```python
from build123d import *

# Parameters (mm, degrees)
SKETCH1_R           = 1.5
BOSS_EXTRUDE1_DEPTH = 3
SCALE1_SCALE        = 0.888888889


with BuildPart() as part:
    # Sketch1 → Boss-Extrude1 (new body)
    with BuildSketch(Plane(origin=(0, 0, 0), x_dir=(1, 0, 0), z_dir=(0, 1, 0))):
        with BuildLine():
            Line((20.893657446, 4), (2.081641936, 4))
            ThreePointArc((2.081641936, 4), (2.861028333, 4.588201733), (3.521749436, 5.30713988))
            ThreePointArc((3.521749436, 5.30713988), (3.405395609, 5.596745198), (3.282888305, 5.883801663))
            ThreePointArc((3.282888305, 5.883801663), (1.93527598, 5.894040025), (0.627094961, 5.57027124))
            ThreePointArc((0.627094961, 5.57027124), (0.366286148, 6.046375), (0.084372603, 6.510293938))
            ThreePointArc((0.084372603, 6.510293938), (1.018855105, 7.48132754), (1.683794586, 8.65351323))
            ThreePointArc((1.683794586, 8.65351323), (1.496450048, 8.903135899), (1.303821399, 9.148703928))
            ThreePointArc((1.303821399, 9.148703928), (-0.000522033, 8.809805691), (-1.180330337, 8.158486898))
            ThreePointArc((-1.180330337, 8.158486898), (-1.555477026, 8.550865528), (-1.947855656, 8.926012217))
            ThreePointArc((-1.947855656, 8.926012217), (-1.296536862, 10.105820521), (-0.957638625, 11.410163953))
            ThreePointArc((-0.957638625, 11.410163953), (-1.203206655, 11.602792602), (-1.452829324, 11.79013714))
            ThreePointArc((-1.452829324, 11.79013714), (-2.625015014, 11.125197659), (-3.596048616, 10.190715157))
            ThreePointArc((-3.596048616, 10.190715157), (-4.059967554, 10.472628702), (-4.536071314, 10.733437515))
            ThreePointArc((-4.536071314, 10.733437515), (-4.212302529, 12.041618533), (-4.222540891, 13.389230859))
            ThreePointArc((-4.222540891, 13.389230859), (-4.509597355, 13.511738163), (-4.799202674, 13.62809199))
            ThreePointArc((-4.799202674, 13.62809199), (-5.759348103, 12.682425791), (-6.455432668, 11.528463019))
            ThreePointArc((-6.455432668, 11.528463019), (-6.976508546, 11.680699536), (-7.503891752, 11.809396783))
            ThreePointArc((-7.503891752, 11.809396783), (-7.529737283, 13.156800143), (-7.888414517, 14.455843809))
            ThreePointArc((-7.888414517, 14.455843809), (-8.197396993, 14.499881098), (-8.507248835, 14.537314892))
            ThreePointArc((-8.507248835, 14.537314892), (-9.18992168, 13.375367565), (-9.563620196, 12.080565177))
            ThreePointArc((-9.563620196, 12.080565177), (-10.106342554, 12.09275), (-10.649064912, 12.080565177))
            ThreePointArc((-10.649064912, 12.080565177), (-11.022763428, 13.375367565), (-11.705436272, 14.537314892))
            ThreePointArc((-11.705436272, 14.537314892), (-12.015288115, 14.499881098), (-12.324270591, 14.455843809))
            ThreePointArc((-12.324270591, 14.455843809), (-12.682947825, 13.156800143), (-12.708793355, 11.809396783))
            ThreePointArc((-12.708793355, 11.809396783), (-13.236176561, 11.680699536), (-13.757252439, 11.528463019))
            ThreePointArc((-13.757252439, 11.528463019), (-14.453337005, 12.682425791), (-15.413482434, 13.62809199))
            ThreePointArc((-15.413482434, 13.62809199), (-15.703087752, 13.511738163), (-15.990144217, 13.389230859))
            ThreePointArc((-15.990144217, 13.389230859), (-16.000382579, 12.041618533), (-15.676613793, 10.733437515))
            ThreePointArc((-15.676613793, 10.733437515), (-16.152717554, 10.472628702), (-16.616636492, 10.190715157))
            ThreePointArc((-16.616636492, 10.190715157), (-17.587670094, 11.125197659), (-18.759855783, 11.79013714))
            ThreePointArc((-18.759855783, 11.79013714), (-19.009478453, 11.602792602), (-19.255046482, 11.410163953))
            ThreePointArc((-19.255046482, 11.410163953), (-18.916148245, 10.105820521), (-18.264829452, 8.926012217))
            ThreePointArc((-18.264829452, 8.926012217), (-18.657208082, 8.550865528), (-19.032354771, 8.158486898))
            ThreePointArc((-19.032354771, 8.158486898), (-20.212163074, 8.809805691), (-21.516506507, 9.148703928))
            ThreePointArc((-21.516506507, 9.148703928), (-21.709135156, 8.903135899), (-21.896479694, 8.65351323))
            ThreePointArc((-21.896479694, 8.65351323), (-21.231540213, 7.48132754), (-20.297057711, 6.510293938))
            ThreePointArc((-20.297057711, 6.510293938), (-20.578971255, 6.046375), (-20.839780068, 5.57027124))
            ThreePointArc((-20.839780068, 5.57027124), (-22.147961087, 5.894040025), (-23.495573413, 5.883801663))
            ThreePointArc((-23.495573413, 5.883801663), (-23.618080717, 5.596745198), (-23.734434544, 5.30713988))
            ThreePointArc((-23.734434544, 5.30713988), (-22.788768345, 4.346994451), (-21.634805572, 3.650909885))
            ThreePointArc((-21.634805572, 3.650909885), (-21.78704209, 3.129834008), (-21.915739337, 2.602450802))
            ThreePointArc((-21.915739337, 2.602450802), (-23.263142697, 2.576605271), (-24.562186363, 2.217928037))
            ThreePointArc((-24.562186363, 2.217928037), (-24.606223651, 1.908945561), (-24.643657446, 1.599093719))
            ThreePointArc((-24.643657446, 1.599093719), (-23.481710119, 0.916420874), (-22.186907731, 0.542722358))
            ThreePointArc((-22.186907731, 0.542722358), (-22.199092554, 0), (-22.186907731, -0.542722358))
            ThreePointArc((-22.186907731, -0.542722358), (-23.481710119, -0.916420874), (-24.643657446, -1.599093719))
            ThreePointArc((-24.643657446, -1.599093719), (-24.606223651, -1.908945561), (-24.562186363, -2.217928037))
            ThreePointArc((-24.562186363, -2.217928037), (-23.263142697, -2.576605271), (-21.915739337, -2.602450802))
            ThreePointArc((-21.915739337, -2.602450802), (-21.78704209, -3.129834008), (-21.634805572, -3.650909885))
            ThreePointArc((-21.634805572, -3.650909885), (-22.788768345, -4.346994451), (-23.734434544, -5.30713988))
            ThreePointArc((-23.734434544, -5.30713988), (-23.618080717, -5.596745198), (-23.495573413, -5.883801663))
            ThreePointArc((-23.495573413, -5.883801663), (-22.147961087, -5.894040025), (-20.839780068, -5.57027124))
            ThreePointArc((-20.839780068, -5.57027124), (-20.578971255, -6.046375), (-20.297057711, -6.510293938))
            ThreePointArc((-20.297057711, -6.510293938), (-21.231540213, -7.48132754), (-21.896479694, -8.65351323))
            ThreePointArc((-21.896479694, -8.65351323), (-21.709135156, -8.903135899), (-21.516506507, -9.148703928))
            ThreePointArc((-21.516506507, -9.148703928), (-20.212163074, -8.809805691), (-19.032354771, -8.158486898))
            ThreePointArc((-19.032354771, -8.158486898), (-18.657208082, -8.550865528), (-18.264829452, -8.926012217))
            ThreePointArc((-18.264829452, -8.926012217), (-18.916148245, -10.105820521), (-19.255046482, -11.410163953))
            ThreePointArc((-19.255046482, -11.410163953), (-19.009478453, -11.602792602), (-18.759855783, -11.79013714))
            ThreePointArc((-18.759855783, -11.79013714), (-17.587670094, -11.125197659), (-16.616636492, -10.190715157))
            ThreePointArc((-16.616636492, -10.190715157), (-16.152717554, -10.472628702), (-15.676613793, -10.733437515))
            ThreePointArc((-15.676613793, -10.733437515), (-16.000382579, -12.041618533), (-15.990144217, -13.389230859))
            ThreePointArc((-15.990144217, -13.389230859), (-15.703087752, -13.511738163), (-15.413482434, -13.62809199))
            ThreePointArc((-15.413482434, -13.62809199), (-14.453337005, -12.682425791), (-13.757252439, -11.528463019))
            ThreePointArc((-13.757252439, -11.528463019), (-13.236176561, -11.680699536), (-12.708793355, -11.809396783))
            ThreePointArc((-12.708793355, -11.809396783), (-12.682947825, -13.156800143), (-12.324270591, -14.455843809))
            ThreePointArc((-12.324270591, -14.455843809), (-12.015288115, -14.499881098), (-11.705436272, -14.537314892))
            ThreePointArc((-11.705436272, -14.537314892), (-11.022763428, -13.375367565), (-10.649064912, -12.080565177))
            ThreePointArc((-10.649064912, -12.080565177), (-10.106342554, -12.09275), (-9.563620196, -12.080565177))
            ThreePointArc((-9.563620196, -12.080565177), (-9.18992168, -13.375367565), (-8.507248835, -14.537314892))
            ThreePointArc((-8.507248835, -14.537314892), (-8.197396993, -14.499881098), (-7.888414517, -14.455843809))
            ThreePointArc((-7.888414517, -14.455843809), (-7.529737283, -13.156800143), (-7.503891752, -11.809396783))
            ThreePointArc((-7.503891752, -11.809396783), (-6.976508546, -11.680699536), (-6.455432668, -11.528463019))
            ThreePointArc((-6.455432668, -11.528463019), (-5.759348103, -12.682425791), (-4.799202674, -13.62809199))
            ThreePointArc((-4.799202674, -13.62809199), (-4.509597355, -13.511738163), (-4.222540891, -13.389230859))
            ThreePointArc((-4.222540891, -13.389230859), (-4.212302529, -12.041618533), (-4.536071314, -10.733437515))
            ThreePointArc((-4.536071314, -10.733437515), (-4.059967554, -10.472628702), (-3.596048616, -10.190715157))
            ThreePointArc((-3.596048616, -10.190715157), (-2.625015014, -11.125197659), (-1.452829324, -11.79013714))
            ThreePointArc((-1.452829324, -11.79013714), (-1.203206655, -11.602792602), (-0.957638625, -11.410163953))
            ThreePointArc((-0.957638625, -11.410163953), (-1.296536862, -10.105820521), (-1.947855656, -8.926012217))
            ThreePointArc((-1.947855656, -8.926012217), (-1.555477026, -8.550865528), (-1.180330337, -8.158486898))
            ThreePointArc((-1.180330337, -8.158486898), (-0.000522033, -8.809805691), (1.303821399, -9.148703928))
            ThreePointArc((1.303821399, -9.148703928), (1.496450048, -8.903135899), (1.683794586, -8.65351323))
            ThreePointArc((1.683794586, -8.65351323), (1.018855105, -7.48132754), (0.084372603, -6.510293938))
            ThreePointArc((0.084372603, -6.510293938), (0.366286148, -6.046375), (0.627094961, -5.57027124))
            ThreePointArc((0.627094961, -5.57027124), (1.93527598, -5.894040025), (3.282888305, -5.883801663))
            ThreePointArc((3.282888305, -5.883801663), (3.405395609, -5.596745198), (3.521749436, -5.30713988))
            ThreePointArc((3.521749436, -5.30713988), (2.861028333, -4.588201733), (2.081641936, -4))
            Line((2.081641936, -4), (20.893657446, -4))
            ThreePointArc((20.893657446, -4), (24.893657446, 0), (20.893657446, 4))
        make_face()
        with Locations(Location((-10.106342554, 0, 0), (0, 0, 270))):
            Circle(SKETCH1_R, mode=Mode.SUBTRACT)
        with Locations(Location((20.893657446, 0, 0), (0, 0, 270))):
            Circle(SKETCH1_R, mode=Mode.SUBTRACT)
    extrude(amount=BOSS_EXTRUDE1_DEPTH)


with BuildPart() as part_1:
    # Scale1: scaled about (-4.801213178, 1.5, 0)
    add(part.part.scale(SCALE1_SCALE).moved(Location((-0.533468131, 0.166666667, 0))))


solid = part_1.part
```
Work out the finished part from the listing and answer in its coordinate system (mm). A direction names the side the tool comes from. Coordinates: 2 decimals unless noted, no trailing zeros. Write each loop counter-clockwise with the first axis right and the second up, starting at its lowest first coordinate (ties: lowest second). Pieces come first, ordered by that corner, then holes.
Q1. A cutting plane is placed at A-A, the plane z = 0. Give the vertices of the cut face in (x, y), then the cut area to 3 significant figures.
Q2. Determine the mould class of faces 5 (the face through (-9.52, 1.48, 10.75)), 6 (the face through (-2.85, 1.48, -9.9)), 7 (the face through (-0.205, 1.481, -5.369)) for opening direction Z: released by +Z, released by -Z, zero draft, split by the parting line, or undercut.
Q3. Which of the six approach directions +Z, -Z, +X, -X, +Y, -Y give full straight-line access (tool end or side, diameter ignored) to faces 1 (the face through (-8.71, 1.48, 11.87)), 2 (the face through (-16.153, 1.481, -9.879)), 3 (the face through (-14.89, 1.48, -9.31)), 4 (the face through (0.362, 1.481, -6.637))?
Q4. Find the intervals of material crossed by line 1 (X direction, y = 1.2, z = 0); line 2 (Z direction, x = 0, y = 2.35); line 3 (X direction, y = 2.05, z = 7.5), in increasing order.
Q5. A cutting plane is placed at B-B, the plane y = 1.4. State how many separate pieces and enclosed holes the cut face has, then the cut area to 3 significant figures.
Q6. This flat-tipped pin is pushed along its axis until it touches: pin 1 Ø1.3 at (x, y) = (8.5, 2) entering from +Z. Where does it stop, or does it pass through?
Findings below:
1. outline: (-20.27, 0.17) - (-10.85, 0.17) - (-10.85, 2.83) - (-20.27, 2.83) - close; (-8.18, 0.17) - (16.71, 0.17) - (16.71, 2.83) - (-8.18, 2.83) - close; (19.37, 0.17) - (21.59, 0.17) - (21.59, 2.83) - (19.37, 2.83) - close
1. area: 97.4 mm2
2. face 5: released by +Z
2. face 6: released by -Z
2. face 7: undercut
3. face 1: +Z, +Y, -Y
3. face 2: -Z, +Y, -Y
3. face 3: +Y, -Y
3. face 4: +X, +Y, -Y
4. line 1: x = -20.27 to -10.85, -8.18 to 16.71, 19.37 to 21.59
4. line 2: z = -8.01 to -6.21, -5 to 5, 6.21 to 8.01
4. line 3: x = -19.91 to -17.83, -17.22 to -1.82, -1.21 to 0.88
5. separate pieces: 1
5. enclosed holes: 2
5. area: 562 mm2
6. pin 1: stops at z = 3.56
